Can you work these out from the model? Positions are in its coordinate system, mm. Face numbers are marked on the shaded views. A direction names the side the tool comes from. Round coordinates to 2 decimals unless told otherwise and drop trailing zeros. Order: outer loops, then holes, each group sorted by start corner. A loop starts at its lowest first (then second) coordinate and runs counter-clockwise, first axis right, second up.
Q1. If we section it at C-C (x = -18.75): Please give me the cut outline in (y, z), plus the area to 3 significant figures.
Q2. For the marked faces 1 and 2, which set-ups out of +Z, -Z, +X, -X, +Y, -Y let a thin tool reach every point of the face, with its end or its side?
Q3. If we section it at B-B (z = 9): Please give me the cut outline in (x, y).
Q4. If we section it at A-A (y = 0): Please give me the cut outline in (x, z), plus the area to 3 significant figures.
Q5. If I drill on line 1 (Z direction, x = -25.5, y = 2); line 2 (X direction, y = -1.75, z = 2.5); line 3 (X direction, y = 3, z = 1), over which ranges is the centre line in solid material (lowest first)?
Q6. Will this pin go through, and if not, where does the flat tip stop? P1, Ø1.5, axis at x = -25.5, y = 1, coming from the +Z side.
from build123d import *

# Parameters (mm, degrees)
F0_R     = 3.25
F1_DEPTH = 13
F0_R_2   = 4.5
F2_DEPTH = 2
F3_R     = 1


with BuildPart() as f1:
    # F0 (on Top) → F1 (new body)
    with BuildSketch(Plane.XY):
        with Locations((-22.529975, 0)):
            Circle(F0_R)
    extrude(amount=F1_DEPTH)

    # F0 (on Top) → F2 (join)
    with BuildSketch(Plane.XY):
        with Locations((-22.529975, 0)):
            Circle(F0_R_2)
        with Locations((-22.529975, 0)):
            Circle(F0_R, mode=Mode.SUBTRACT)
        with Locations((-22.529975, 0)):
            Circle(F0_R)
    extrude(amount=-F2_DEPTH)

    # F3
    f3_edges = [f1.edges().sort_by_distance(p)[0] for p in [
        (-25.779975, 0, 13),
    ]]
    fillet(f3_edges, radius=F3_R)


solid = f1.part
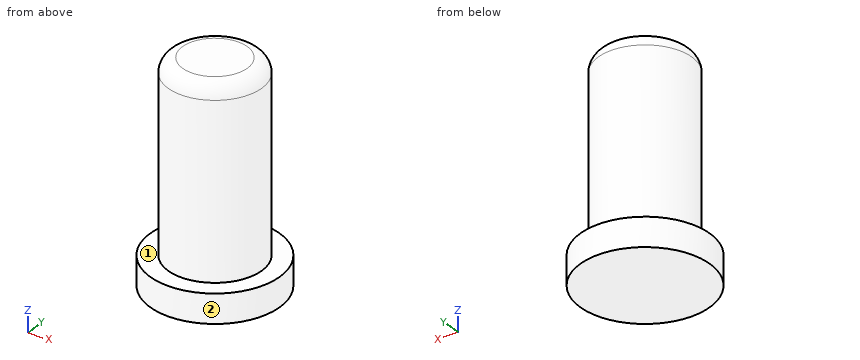
Solution:
1. outline: (-2.44, -2) - (2.44, -2) - (2.44, 0) - (-2.44, 0) - close
1. area: 9.77 mm2
2. face 1: +Z
2. face 2: +Z, -Z
3. outline: circle Ø6.5 at (-22.53, 0)
4. outline: (-27.03, -2) - (-18.03, -2) - (-18.03, 0) - (-19.28, 0) - (-19.28, 12) arc R1 ccw to (-20.28, 13) - (-24.78, 13) arc R1 ccw to (-25.78, 12) - (-25.78, 0) - (-27.03, 0) - close
4. area: 102 mm2
5. line 1: z = -2 to 0
5. line 2: x = -25.27 to -19.79
5. line 3: x = -23.78 to -21.28
6. P1: stops at z = 12.99
